Can you work these out from the model? Positions are in its coordinate system, mm. Face numbers are marked on the shaded views. A direction names the side the tool comes from. Round coordinates to 2 decimals unless told otherwise and drop trailing zeros. Order: outer loops, then holes, each group sorted by start corner. A loop starts at its lowest first (then second) coordinate and runs counter-clockwise, first axis right, second up.
Q1. If we section it at C-C (x = 15): Please give me the cut outline in (y, z), plus the area to 3 significant figures.
Q2. For the marked faces 4 and 5, which set-ups out of +Z, -Z, +X, -X, +Y, -Y let a thin tool reach every point of the face, with its end or its side?
Q3. If I drill on line 1 (Y direction, x = 19.5, z = 45.5); line 2 (Z direction, x = 13.5, y = -6); line 3 (X direction, y = 1.5, z = 44), over which ranges is the centre line in solid material (lowest first)?
Q4. We'd pull the mould along Y, two halves only. Please class the marked faces 1, 2 and 3: pulls with the +Y half, pulls with the -Y half, needs draft (parallel to the pull), parting line crosses it, or undercut.
Q5. If we section it at A-A (x = 31.5): Please give me the cut outline in (y, z), plus the area to 3 significant figures.
Q6. Will these pins go through, and if not, where does the flat tip stop? P1, Ø12, axis at x = 22, y = -40, coming from the +Z side; P2, Ø4.5, axis at x = 20, z = 53, coming from the -Y side; P3, Ø7, axis at y = -30.5, z = 48.5, coming from the -X side; P4, Ø7, axis at x = 31.5, z = 50.5, coming from the -Y side.
Q7. If we section it at B-B (y = -40.5): Please give me the cut outline in (x, z).
from build123d import *

# Parameters (mm, degrees)
SKETCH1_W           = 159
SKETCH1_H           = 99
BOSS_EXTRUDE1_DEPTH = 42
SKETCH2_W           = 14.5
SKETCH2_H           = 97.8
CUT_EXTRUDE1_DEPTH  = 40.8
SKETCH3_W           = 14.5
SKETCH3_H           = 68.5
BOSS_EXTRUDE2_DEPTH = 16
SKETCH5_R           = 1.5
CUT_EXTRUDE2_DEPTH  = 5


with BuildPart() as part:
    # Sketch1 → Boss-Extrude1 (new body)
    with BuildSketch(Plane(origin=(0, 0, 0), x_dir=(0, 0, -1), z_dir=(1, 0, 0))):
        with Locations((22.6575, -29.7045)):
            Rectangle(SKETCH1_W, SKETCH1_H)
    extrude(amount=BOSS_EXTRUDE1_DEPTH)

    # Sketch2 → Cut-Extrude1 (cut)
    with BuildSketch(Plane.ZY):
        with Locations((49.5925, -30.3045)):
            Rectangle(SKETCH2_W, SKETCH2_H)
    extrude(amount=-CUT_EXTRUDE1_DEPTH, mode=Mode.SUBTRACT)

    # Sketch3 → Boss-Extrude2 (add)
    with BuildSketch(Plane.ZY.offset(-40.8)):
        with Locations((49.5925, -32.9545)):
            Rectangle(SKETCH3_W, SKETCH3_H)
    extrude(amount=BOSS_EXTRUDE2_DEPTH)

    # Sketch5 → Cut-Extrude2 (cut)
    with BuildSketch(Plane(origin=(42, 0, 0), x_dir=(0, 0, -1), z_dir=(1, 0, 0))):
        with Locations((-32.3425, -12.7045)):
            Circle(SKETCH5_R)
        with Locations((59.009480141, -12.7045)):
            Circle(SKETCH5_R)
    extrude(amount=-CUT_EXTRUDE2_DEPTH, mode=Mode.SUBTRACT)


solid = part.part
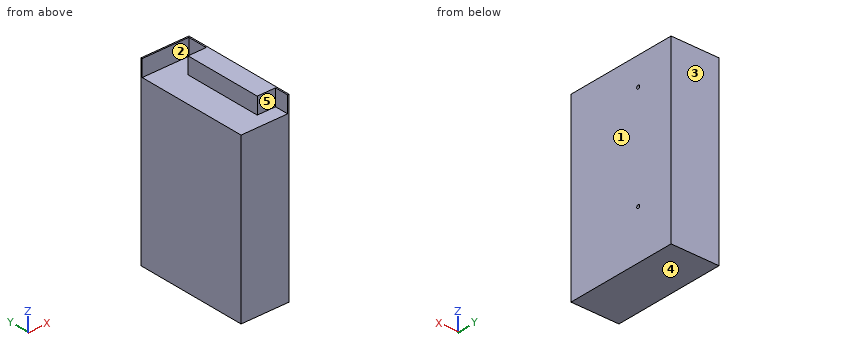
Solution:
1. outline: (-79.2, -102.16) - (19.8, -102.16) - (19.8, 56.84) - (18.6, 56.84) - (18.6, 42.34) - (-79.2, 42.34) - close
1. area: 14,300 mm2
2. face 4: -Z, +X, -X, +Y, -Y
2. face 5: +Z, -X, -Y
3. line 1: y = 18.6 to 19.8
3. line 2: z = -102.16 to 42.34
3. line 3: x = 40.8 to 42
4. face 1: needs draft
4. face 2: undercut
4. face 3: pulls with the +Y half
5. outline: (-79.2, -102.16) - (19.8, -102.16) - (19.8, 56.84) - (18.6, 56.84) - (18.6, 42.34) - (1.3, 42.34) - (1.3, 56.84) - (-67.2, 56.84) - (-67.2, 42.34) - (-79.2, 42.34) - close
5. area: 15,300 mm2
6. P1: stops at z = 56.84
6. P2: stops at y = 18.6
6. P3: stops at x = 24.8
6. P4: stops at y = -67.2
7. outline: (0, -102.16) - (42, -102.16) - (42, 56.84) - (24.8, 56.84) - (24.8, 42.34) - (0, 42.34) - close
